Read the model definition and answer for the solid it produces. Units are mm, in the model's axes. Face numbers are marked on the shaded views. A direction names the side the tool comes from. Round coordinates to 2 decimals unless told otherwise and drop trailing zeros. Order: outer loops, then holes, each group sorted by start corner. A loop starts at its lowest first (then second) coordinate and runs counter-clockwise, first axis right, second up. Notation, with made-up numbers: M -15,53 L -6,53 A23 ccw -6,91 Z; hole C 39,43.5 d3. An arc over 180 degrees is marked long. Answer as CSV lines item,"result".
```python
from build123d import *

# Parameters (mm, degrees)
SKETCH1_W                 = 38.1
SKETCH1_H                 = 50.8
BOSS_EXTRUDE1_DEPTH       = 25.4
CUT_EXTRUDE1_DEPTH        = 25.4
SKETCH3_W                 = 31.75
SKETCH3_H                 = 31.75
CUT_EXTRUDE2_DEPTH        = 21.59
SKETCH5_W                 = 12.7
SKETCH5_H                 = 12.7
CUT_EXTRUDE3_DEPTH        = 3.81
SKETCH4_W                 = 12.7
SKETCH4_H                 = 25.4
CUT_EXTRUDE4_DEPTH        = 3.175
SKETCH6_W                 = 6.35
SKETCH6_H                 = 5.08
SKETCH6_W_2               = 31.75
BOSS_EXTRUDE2_DEPTH       = 25.4
CUT_EXTRUDE5_START        = -25.4
SKETCH7_R                 = 1.7145
CUT_EXTRUDE5_DEPTH        = 25.4
SKETCH8_R                 = 3.175
CUT_EXTRUDE6_DEPTH        = 18.796
CUT_EXTRUDE7_START        = -25.4
SKETCH9_R                 = 3.175
CUT_EXTRUDE7_DEPTH        = 25.4
SKETCH10_R                = 4.826
SKETCH10_R_2              = 3.175
SKETCH10_R_3              = 4.7625
BOSS_EXTRUDE3_DEPTH       = 25.4
SKETCH11_R                = 3.175
BOSS_EXTRUDE4_DEPTH       = 25.4
SKETCH12_R                = 3.175
SKETCH12_R_2              = 1.651
BOSS_EXTRUDE5_DEPTH       = 5
BOSS_EXTRUDE6_DEPTH       = 25.4
BOSS_EXTRUDE7_DEPTH       = 25.4
SKETCH15_W                = 25.4
SKETCH15_H                = 38.1
BOSS_EXTRUDE8_DEPTH       = 5.08
CUT_EXTRUDE9_START        = -21.59
SKETCH16_W                = 9.228
SKETCH16_H                = 3.577281452
CUT_EXTRUDE9_DEPTH        = 21.59
FILLET1_R                 = 30.48
FILLET2_R                 = 2.54
CUT_EXTRUDE10_START       = -21.59
SKETCH17_W                = 31.75
SKETCH17_H                = 27.158947133
CUT_EXTRUDE10_DEPTH       = 21.59
CUT_EXTRUDE11_START       = -21.59
SKETCH18_W                = 31.75
SKETCH18_H                = 1.235371837
CUT_EXTRUDE11_DEPTH       = 21.59
SKETCH19_W                = 5.08
SKETCH19_H                = 28.39431897
BOSS_EXTRUDE9_DEPTH       = 21.59
SKETCH20_R                = 1.651
CUT_EXTRUDE12_DEPTH       = 25.4
BOSS_EXTRUDE10_START      = -3.81
BOSS_EXTRUDE10_DEPTH      = 3.81
SKETCH23_W                = 21.59
SKETCH23_H                = 13.188947133
CUT_EXTRUDE13_DEPTH       = 3.81
BOSS_EXTRUDE13_DEPTH      = 21.59
BOSS_EXTRUDE13_DEPTH_BACK = 3.81
SKETCH24_W                = 1.27
SKETCH24_H                = 28.39431897
SKETCH25_W                = 12.7
SKETCH25_H                = 2.686052867
BOSS_EXTRUDE14_DEPTH      = 31.75


with BuildPart() as part:
    # Sketch1 → Boss-Extrude1 (new body)
    with BuildSketch(Plane.YZ):
        with Locations((19.05, 25.4)):
            Rectangle(SKETCH1_W, SKETCH1_H)
    extrude(amount=BOSS_EXTRUDE1_DEPTH)

    # Sketch2 → Cut-Extrude1 (cut)
    with BuildSketch(Plane.YZ.offset(25.4)):
        Polygon((13.3985, 12.7), (24.7015, 12.7), (24.7015, 8.250084788), (22.352, 8.250084788), (22.352, 0), (15.748, 0), (15.748, 8.250084788), (13.3985, 8.250084788), align=None)
    extrude(amount=-CUT_EXTRUDE1_DEPTH, mode=Mode.SUBTRACT)

    # Sketch3 → Cut-Extrude2 (cut)
    with BuildSketch(Plane.YZ.offset(25.4)):
        with Locations((19.05, 31.75)):
            Rectangle(SKETCH3_W, SKETCH3_H)
    extrude(amount=-CUT_EXTRUDE2_DEPTH, mode=Mode.SUBTRACT)

    # Sketch5 → Cut-Extrude3 (cut)
    with BuildSketch(Plane(origin=(0, 0, 0), x_dir=(0, -1, 0), z_dir=(-1, 0, 0))):
        with Locations((-12.7, 22.225)):
            Rectangle(SKETCH5_W, SKETCH5_H)
    extrude(amount=-CUT_EXTRUDE3_DEPTH, mode=Mode.SUBTRACT)

    # Sketch4 → Cut-Extrude4 (cut)
    with BuildSketch(Plane.XY.offset(15.875)):
        with Locations((10.16, 19.05)):
            Rectangle(SKETCH4_W, SKETCH4_H)
    extrude(amount=-CUT_EXTRUDE4_DEPTH, mode=Mode.SUBTRACT)

    # Sketch6 → Boss-Extrude2 (add)
    with BuildSketch(Plane.YZ.offset(25.4)):
        with Locations((6.35, 18.415)):
            Rectangle(SKETCH6_W, SKETCH6_H)
        with Locations((31.75, 18.415)):
            Rectangle(SKETCH6_W, SKETCH6_H)
        with Locations((19.05, 45.085)):
            Rectangle(SKETCH6_W_2, SKETCH6_H)
    extrude(amount=-BOSS_EXTRUDE2_DEPTH)

    # Sketch7 → Cut-Extrude5 (cut)
    with BuildSketch(Plane(origin=(0, 0, 0), x_dir=(0, -1, 0), z_dir=(-1, 0, 0)).offset(CUT_EXTRUDE5_START)):
        with Locations(Location((-20.066, 46.303766696, 0), (0, 0, 90))):
            Circle(SKETCH7_R)
        with Locations(Location((-5.334, 46.303766696, 0), (0, 0, 90))):
            Circle(SKETCH7_R)
        with Locations(Location((-4.496233304, 16.002, 0), (0, 0, 90))):
            Circle(SKETCH7_R)
        with Locations(Location((-20.903766696, 16.002, 0), (0, 0, 90))):
            Circle(SKETCH7_R)
    extrude(amount=CUT_EXTRUDE5_DEPTH, mode=Mode.SUBTRACT)

    # Sketch8 → Cut-Extrude6 (cut)
    with BuildSketch(Plane(origin=(0, 0, 0), x_dir=(0, -1, 0), z_dir=(-1, 0, 0))):
        with Locations(Location((-20.066, 46.303766696, 0), (0, 0, 90))):
            Circle(SKETCH8_R)
        with Locations(Location((-5.334, 46.303766696, 0), (0, 0, 90))):
            Circle(SKETCH8_R)
        with Locations(Location((-4.496233304, 16.002, 0), (0, 0, 90))):
            Circle(SKETCH8_R)
        with Locations((-20.903766696, 16.002)):
            Circle(SKETCH8_R)
    extrude(amount=-CUT_EXTRUDE6_DEPTH, mode=Mode.SUBTRACT)

    # Sketch9 → Cut-Extrude7 (cut)
    with BuildSketch(Plane(origin=(0, 0, 0), x_dir=(0, -1, 0), z_dir=(-1, 0, 0)).offset(CUT_EXTRUDE7_START)):
        with Locations(Location((-20.066, 37.819300087, 0), (0, 0, 90))):
            Circle(SKETCH9_R)
        with Locations((-5.334, 24.054233304)):
            Circle(SKETCH9_R)
    extrude(amount=CUT_EXTRUDE7_DEPTH, mode=Mode.SUBTRACT)

    # Sketch10 → Boss-Extrude3 (add)
    # profile 1 of 2: a face of its own
    with BuildSketch(Plane.YZ.offset(25.4)):
        with Locations((5.334, 24.054233304)):
            Circle(SKETCH10_R)
        with Locations(Location((5.334, 24.054233304, 0), (0, 0, 90))):
            Circle(SKETCH10_R_2, mode=Mode.SUBTRACT)
    # profile 2 of 2: a face of its own
    with BuildSketch(Plane.YZ.offset(25.4)):
        with Locations((20.066, 37.819300087)):
            Circle(SKETCH10_R_3)
        with Locations(Location((20.066, 37.819300087, 0), (0, 0, 90))):
            Circle(SKETCH10_R_2, mode=Mode.SUBTRACT)
    extrude(amount=-BOSS_EXTRUDE3_DEPTH)

    # Sketch11 → Boss-Extrude4 (add)
    with BuildSketch(Plane(origin=(0, 0, 0), x_dir=(0, -1, 0), z_dir=(-1, 0, 0))):
        with Locations(Location((-20.903766696, 16.002, 0), (0, 0, 357.707557224))):
            Circle(SKETCH11_R)
        with Locations((-4.496233304, 16.002)):
            Circle(SKETCH11_R)
        with Locations((-20.066, 46.303766696)):
            Circle(SKETCH11_R)
        with Locations((-5.334, 46.303766696)):
            Circle(SKETCH11_R)
    extrude(amount=-BOSS_EXTRUDE4_DEPTH)

    # Sketch12 → Boss-Extrude5 (add)
    # profile 1 of 2: a face of its own
    with BuildSketch(Plane.YZ.offset(25.4)):
        with Locations(Location((5.334, 24.054233304, 0), (0, 0, 90))):
            Circle(SKETCH12_R)
        with Locations(Location((5.334, 24.054233304, 0), (0, 0, 270))):
            Circle(SKETCH12_R_2, mode=Mode.SUBTRACT)
    # profile 2 of 2: a face of its own
    with BuildSketch(Plane.YZ.offset(25.4)):
        with Locations(Location((20.066, 37.819300087, 0), (0, 0, 90))):
            Circle(SKETCH12_R)
        with Locations(Location((20.066, 37.819300087, 0), (0, 0, 270))):
            Circle(SKETCH12_R_2, mode=Mode.SUBTRACT)
    extrude(amount=-BOSS_EXTRUDE5_DEPTH)

    # Sketch13 → Boss-Extrude6 (add)
    with BuildSketch(Plane.YZ.offset(25.4)):
        with BuildLine():
            Line((22.225, 42.064311895), (22.225, 42.545))
            Line((22.225, 42.545), (20.656903194, 42.545))
            ThreePointArc((20.656903194, 42.545), (21.461799827, 42.372666874), (22.225, 42.064311895))
        make_face()
    extrude(amount=-BOSS_EXTRUDE6_DEPTH)

    # Sketch14 → Boss-Extrude7 (add)
    with BuildSketch(Plane.YZ.offset(25.4)):
        with BuildLine():
            Line((19.475096806, 42.545), (15.3035, 42.545))
            Line((15.3035, 42.545), (15.3035, 37.819300087))
            ThreePointArc((15.3035, 37.819300087), (16.495595071, 40.971063862), (19.475096806, 42.545))
        make_face()
    extrude(amount=-BOSS_EXTRUDE7_DEPTH)

    # Sketch15 → Boss-Extrude8 (add)
    with BuildSketch(Plane.XY.offset(50.8)):
        with Locations((12.7, 19.05)):
            Rectangle(SKETCH15_W, SKETCH15_H)
    extrude(amount=BOSS_EXTRUDE8_DEPTH)

    # Sketch16 → Cut-Extrude9 (cut)
    with BuildSketch(Plane.YZ.offset(25.4).offset(CUT_EXTRUDE9_START)):
        with Locations((12.700000043, 41.880359274)):
            Rectangle(SKETCH16_W, SKETCH16_H)
    extrude(amount=CUT_EXTRUDE9_DEPTH, mode=Mode.SUBTRACT)

    # Fillet1
    # the kernel refuses this fillet: 30.48 mm, written as the material it takes off along each edge
    with BuildSketch(Plane(origin=(3.81, 15.3035, 40.091718548), x_dir=(0, 0, -1), z_dir=(1, 0, 0))) as fillet1_piece_1:
        with BuildLine():
            CenterArc((10.886595988, 30.48), FILLET1_R, 249.07339313, 20.92660687)
            Line((0, 2.010500043), (0, 0))
            Line((0, 0), (10.886595988, 0))
        make_face()
    extrude(amount=48.806489969, mode=Mode.SUBTRACT)

    # Fillet2
    fillet2_edges = [part.edges().sort_by_distance(p)[0] for p in [
        (14.605, 15.945995831, 35.430373154),
    ]]
    fillet(fillet2_edges, radius=FILLET2_R)

    # Sketch17 → Cut-Extrude10 (cut)
    with BuildSketch(Plane.YZ.offset(25.4).offset(CUT_EXTRUDE10_START)):
        with Locations((19.05, 28.965526434)):
            Rectangle(SKETCH17_W, SKETCH17_H)
    extrude(amount=CUT_EXTRUDE10_DEPTH, mode=Mode.SUBTRACT)

    # Sketch18 → Cut-Extrude11 (cut)
    with BuildSketch(Plane.YZ.offset(25.4).offset(CUT_EXTRUDE11_START)):
        with Locations((19.05, 43.162685919)):
            Rectangle(SKETCH18_W, SKETCH18_H)
    extrude(amount=CUT_EXTRUDE11_DEPTH, mode=Mode.SUBTRACT)

    # Sketch19 → Boss-Extrude9 (add)
    with BuildSketch(Plane.YZ.offset(3.81)):
        with Locations((5.715, 29.583212352)):
            Rectangle(SKETCH19_W, SKETCH19_H)
        with Locations((32.385, 29.583212352)):
            Rectangle(SKETCH19_W, SKETCH19_H)
    extrude(amount=BOSS_EXTRUDE9_DEPTH)

    # Sketch20 → Cut-Extrude12 (cut)
    with BuildSketch(Plane.YZ.offset(25.4)):
        with Locations(Location((4.7625, 26.67, 0), (0, 0, 270))):
            Circle(SKETCH20_R)
        with Locations(Location((33.3375, 26.67, 0), (0, 0, 270))):
            Circle(SKETCH20_R)
    extrude(amount=-CUT_EXTRUDE12_DEPTH, mode=Mode.SUBTRACT)

    # Sketch22 → Boss-Extrude10 (add)
    with BuildSketch(Plane(origin=(0, 0, 0), x_dir=(0, -1, 0), z_dir=(-1, 0, 0)).offset(BOSS_EXTRUDE10_START)):
        with BuildLine():
            Line((-7.023066157, 28.575), (-8.255, 28.575))
            Line((-8.255, 28.575), (-8.255, 27.895852104))
            ThreePointArc((-8.255, 27.895852104), (-7.663911578, 28.280554168), (-7.023066157, 28.575))
        make_face()
        with BuildLine():
            ThreePointArc((-6.367681938, 27.056253732), (-5.182460289, 25.073305178), (-3.175, 26.216519295))
            ThreePointArc((-3.175, 26.216519295), (-3.157324346, 26.283720153), (-3.142492042, 26.351605253))
            ThreePointArc((-3.142492042, 26.351605253), (-6.011696572, 20.952402819), (-6.367681938, 27.056253732))
        make_face()
    extrude(amount=BOSS_EXTRUDE10_DEPTH)

    # Sketch23 → Cut-Extrude13 (cut)
    with BuildSketch(Plane.YZ.offset(3.81)):
        with Locations((19.05, 21.980526434)):
            Rectangle(SKETCH23_W, SKETCH23_H)
    extrude(amount=-CUT_EXTRUDE13_DEPTH, mode=Mode.SUBTRACT)

    # Sketch24 → Boss-Extrude13 (add, two sides: drawn at the far end of the back side and taken through both)
    with BuildSketch(Plane.YZ.offset(3.81).offset(-BOSS_EXTRUDE13_DEPTH_BACK)):
        with Locations((29.21, 29.583212352)):
            Rectangle(SKETCH24_W, SKETCH24_H)
        with Locations((8.89, 29.583212352)):
            Rectangle(SKETCH24_W, SKETCH24_H)
    extrude(amount=BOSS_EXTRUDE13_DEPTH + BOSS_EXTRUDE13_DEPTH_BACK)

    # Sketch25 → Boss-Extrude14 (add)
    with BuildSketch(Plane.XZ.offset(-31.75)):
        with Locations((10.16, 14.043026433)):
            Rectangle(SKETCH25_W, SKETCH25_H)
    extrude(amount=BOSS_EXTRUDE14_DEPTH)


solid = part.part
```
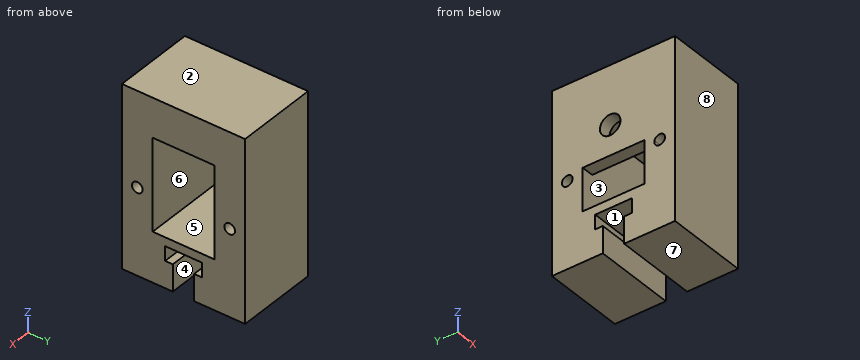
Item 1: A tool of negligible diameter and unlimited length cuts with its end or side. For the marked faces 1, 2, 3 and 4, from which of +Z, -Z, +X, -X, +Y, -Y can it reach the whole face along a straight path? Write none if from no direction.
Ans:
face 1,"+X, -X"
face 2,"+Z, +X, -X, +Y, -Y"
face 3,"+X"
face 4,"-Z, +X, -X"
Item 2: A cutting plane is placed at D-D, the plane x = 8. Give the number of separate pieces and of enclosed holes in the cut face, and give its area (3 significant figures).
Ans:
separate pieces,"1"
enclosed holes,"3"
area,"1,460 mm2"
Item 3: Find the intervals of material crossed by probe 1 along Y at (x, z) = (16.5, 26.67) (1 decimal); probe 2 along Z at (x, y) = (2, 14.5) (3 decimals); probe 3 along Y at (x, z) = (20, 5), in increasing order. Write a range as [from, to].
Ans:
probe 1,"[0, 3.1], [6.4, 9.5], [28.6, 31.7], [35, 38.1]"
probe 2,"[0, 8.25], [12.7, 15.386], [28.575, 55.88]"
probe 3,"[0, 15.75], [22.35, 38.1]"
Item 4: A cutting plane is placed at B-B, the plane y = 11. Determine the outline of the cut face in (x, z) (3 decimals).
Ans:
outline,"M 0,0 L 25.4,0 L 25.4,15.386 L 0,15.386 Z; M 0,28.575 L 3.81,28.575 L 3.81,43.78 L 25.4,43.78 L 25.4,55.88 L 0,55.88 Z"
Item 5: Flat-ended cylindrical pins translate along their axes: pin 1 (3.5 mm diameter, centred on x = 16, y = 20, fed in from -Z); pin 2 (2 mm diameter, centred on y = 4.76, z = 26.67, fed in from +X); pin 3 (10 mm diameter, centred on y = 20.07, z = 37.82, fed in from -X); pin 4 (7.5 mm diameter, centred on y = 15, z = 34, fed in from +X). Find the tip coordinate at first contact, or state that the pin passes through.
Ans:
pin 1,"z = 12.7"
pin 2,"through"
pin 3,"x = 0"
pin 4,"x = 3.81"
Item 6: A cutting plane is placed at A-A, the plane z = 7. Determine the outline of the cut face in (x, y).
Ans:
outline,"M 0,0 L 25.4,0 L 25.4,15.75 L 0,15.75 Z; M 0,22.35 L 25.4,22.35 L 25.4,38.1 L 0,38.1 Z"
Item 7: Determine the mould class of the marked faces 5, 6, 7 and 8 for opening direction Z: +Z half, -Z half, draft (parallel to the pull), parting line (faces both ways), or undercut.
Ans:
face 5,"undercut"
face 6,"undercut"
face 7,"-Z half"
face 8,"draft"
Item 8: A cutting plane is placed at C-C, the plane y = 21. Determine the outline of the cut face in (x, z) (3 decimals).
Ans:
outline,"M 0,12.7 L 25.4,12.7 L 25.4,15.386 L 0,15.386 Z; M 0,28.575 L 3.81,28.575 L 3.81,34.785 L 0,34.785 Z; M 0,40.854 L 3.81,40.854 L 3.81,43.78 L 25.4,43.78 L 25.4,55.88 L 0,55.88 Z"
